Input: dimensioned drawing with shaded views. Units: mm. Origin: part minimum x, y, z. A direction names the side the tool comes from. Give positions to 0.01 mm unless a question says otherwise; leave off trailing zeros. Loops run counter-clockwise (first coordinate to the right, second up) from the corner with the lowest first, then second, coordinate; pieces in that order, holes last. Notation, with made-up numbers: (3, 63.5) -> (28, 63.5) arc R11 ccw to (28, 80.5) -> close; hole circle Ø3 at (-37.75, 59). An arc over 180 degrees is marked (long way). Answer as a JSON object with one key per item and string values.
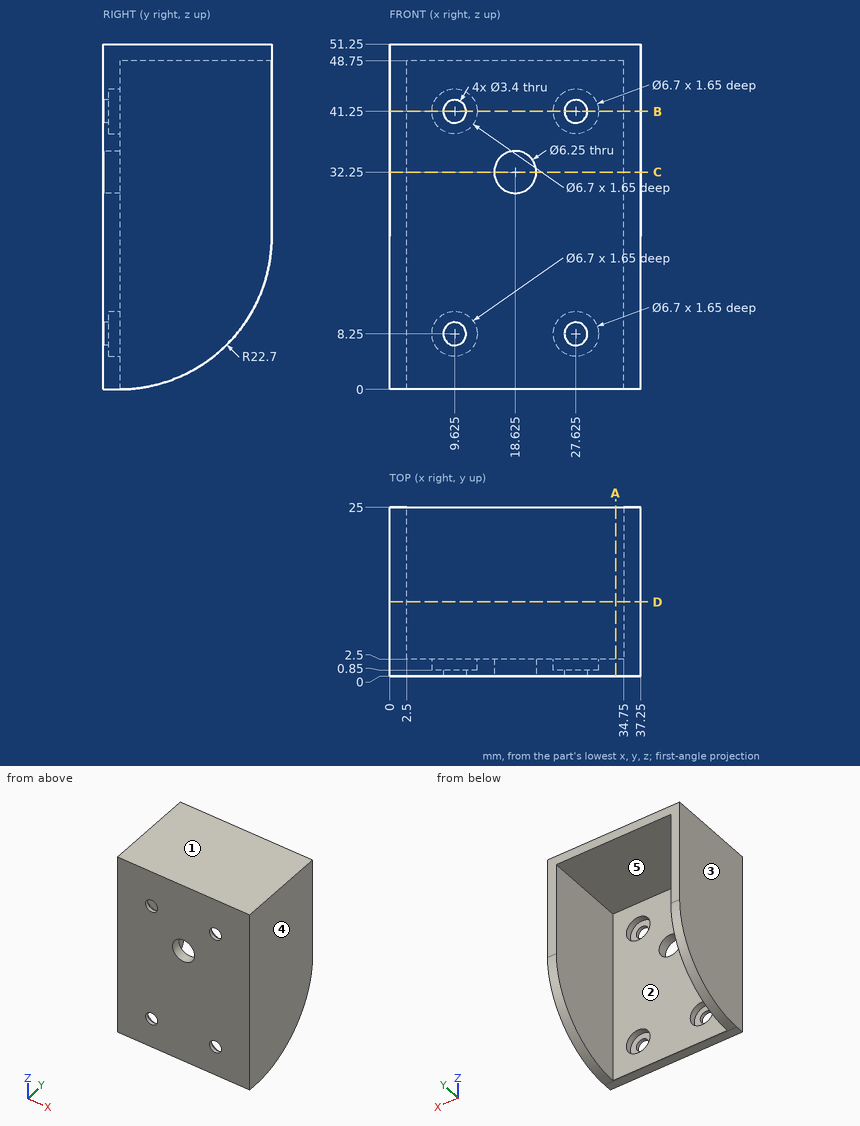
Q1. Draft query along X for the marked faces 1, 2 and 3. Return one class per face: +X half, -X half, draft (parallel to the pull), parting line (faces both ways), or undercut.
Evaluation:
{"face 1": "draft", "face 2": "undercut", "face 3": "-X half"}
Q2. Access query for the marked faces 4 and 5. Directions: +Z, -Z, +X, -X, +Y, -Y. A direction counts if a zero-diameter tool reaches every point of the face in a straight line with its end or side. Return the directions, or none.
Evaluation:
{"face 4": "+Z, -Z, +X, +Y, -Y", "face 5": "-Z, +Y"}
Q3. Section C-C, the plane z = 32.25. Return the cut outline in (x, y).
Evaluation:
{"outline": "(0, 0) -> (15.5, 0) -> (15.5, 2.5) -> (2.5, 2.5) -> (2.5, 25) -> (0, 25) -> close; (21.75, 0) -> (37.25, 0) -> (37.25, 25) -> (34.75, 25) -> (34.75, 2.5) -> (21.75, 2.5) -> close"}
Q4. Section B-B, the plane z = 41.25. Return the cut outline in (x, y) (3 decimals), then the cut area to 3 significant figures.
Evaluation:
{"outline": "(0, 0) -> (7.925, 0) -> (7.925, 0.85) -> (6.275, 0.85) -> (6.275, 2.5) -> (2.5, 2.5) -> (2.5, 25) -> (0, 25) -> close; (11.325, 0) -> (25.925, 0) -> (25.925, 0.85) -> (24.275, 0.85) -> (24.275, 2.5) -> (12.975, 2.5) -> (12.975, 0.85) -> (11.325, 0.85) -> close; (29.325, 0) -> (37.25, 0) -> (37.25, 25) -> (34.75, 25) -> (34.75, 2.5) -> (30.975, 2.5) -> (30.975, 0.85) -> (29.325, 0.85) -> close", "area": "178 mm2"}
Q5. Section D-D, the plane y = 11. Return the cut outline in (x, z).
Evaluation:
{"outline": "(0, 1.73) -> (2.5, 1.73) -> (2.5, 48.75) -> (34.75, 48.75) -> (34.75, 1.73) -> (37.25, 1.73) -> (37.25, 51.25) -> (0, 51.25) -> close"}
Q6. Pin query (flat end, axial travel): pin 1 (7.5 mm diameter, centred on x = 27.625, z = 8.25, fed in from +Y); pin 2 (1.5 mm diameter, centred on x = 7, y = 6, fed in from -Z); pin 3 (3.5 mm diameter, centred on x = 26.5, z = 8.5, fed in from +Y). Return the tip coordinate at first contact, or that it passes through.
Evaluation:
{"pin 1": "stops at y = 2.5", "pin 2": "stops at z = 48.75", "pin 3": "stops at y = 0.85"}
Q7. Section A-A, the plane x = 33.5. Return the cut outline in (y, z).
Evaluation:
{"outline": "(0, 0) -> (2.3, 0) arc R22.7 ccw to (2.5, 0) -> (2.5, 48.75) -> (25, 48.75) -> (25, 51.25) -> (0, 51.25) -> close"}
Q8. Ray query, line 1 along X through (y, z) = (15, 4); line 2 along Z through (x, y) = (31, 20); line 3 along Y through (x, z) = (9, 10). Return the intervals inside material, ascending.
Evaluation:
{"line 1": "x = 0 to 2.5, 34.75 to 37.25", "line 2": "z = 48.75 to 51.25", "line 3": "y = 0 to 0.85"}
